The model under review builds one solid part; all positions refer to its coordinate system, in mm. A direction names the side the tool comes from. Coordinates: 2 decimals unless noted, no trailing zeros. Order: outer loops, then holes, each group sorted by start corner. A loop starts at its lowest first (then second) coordinate and runs counter-clockwise, first axis right, second up.
```python
from build123d import *

# Parameters (mm, degrees)
EXTRUDE_1_DEPTH     = 20
SKETCH_2_R          = 1.5
CUT_EXTRUDE_1_DEPTH = 4
SKETCH_3_R          = 2
CUT_EXTRUDE_2_DEPTH = 19
SKETCH_4_W          = 20
SKETCH_4_H          = 15
CUT_EXTRUDE_3_DEPTH = 1
SKETCH_5_W          = 20
SKETCH_5_H          = 23
CUT_EXTRUDE_4_DEPTH = 1


with BuildPart() as part:
    # 草图1 → 凸台-拉伸1 (new body)
    with BuildSketch(Plane(origin=(0, 0, 0), x_dir=(0, 0, -1), z_dir=(1, 0, 0))):
        Polygon((0, 0), (0, 25), (3, 25), (3, 3), (18, 3), (18, 0), align=None)
    extrude(amount=EXTRUDE_1_DEPTH)

    # 草图2 → 切除-拉伸1 (cut, through all)
    with BuildSketch(Plane(origin=(0, 3, 0), x_dir=(1, 0, 0), z_dir=(0, 1, 0))):
        with Locations((5.5, 8)):
            Circle(SKETCH_2_R)
        with Locations((14.5, 8)):
            Circle(SKETCH_2_R)
    extrude(amount=-CUT_EXTRUDE_1_DEPTH, mode=Mode.SUBTRACT)

    # 草图3 → 切除-拉伸2 (cut, through all)
    with BuildSketch(Plane.XY):
        with Locations((10, 16)):
            Circle(SKETCH_3_R)
    extrude(amount=-CUT_EXTRUDE_2_DEPTH, mode=Mode.SUBTRACT)

    # 草图4 → 切除-拉伸3 (cut)
    with BuildSketch(Plane(origin=(0, 3, 0), x_dir=(1, 0, 0), z_dir=(0, 1, 0))):
        with Locations((10, 10.5)):
            Rectangle(SKETCH_4_W, SKETCH_4_H)
    extrude(amount=-CUT_EXTRUDE_3_DEPTH, mode=Mode.SUBTRACT)

    # 草图5 → 切除-拉伸4 (cut)
    with BuildSketch(Plane(origin=(0, 0, -3), x_dir=(-1, 0, 0), z_dir=(0, 0, -1))):
        with Locations((-10, 13.5)):
            Rectangle(SKETCH_5_W, SKETCH_5_H)
    extrude(amount=-CUT_EXTRUDE_4_DEPTH, mode=Mode.SUBTRACT)


solid = part.part
```
(1) We need section A-A, the plane x = 14.5. Write out the cut boundary in (y, z), and give its area (3 significant figures).
A:
outline: (0, -18) - (2, -18) - (2, -9.5) - (0, -9.5) - close; (0, -6.5) - (2, -6.5) - (2, -2) - (25, -2) - (25, 0) - (0, 0) - close
area: 76.0 mm2
(2) We need section C-C, the plane y = 16. Write out the cut boundary in (x, z).
A:
outline: (0, -2) - (8, -2) - (8, 0) - (0, 0) - close; (12, -2) - (20, -2) - (20, 0) - (12, 0) - close
(3) Machinability: for faces 5 (the face through (10.1, 13.7, -2)), 6 (the face through (20, 7.9, -1.7)), which of the approach directions +Z, -Z, +X, -X, +Y, -Y give a long, thin tool a straight path to every point of the face, cutting with its end or side? Answer none if there is none.
A:
face 5: -Z, +X, -X, +Y
face 6: +Z, -Z, +X, +Y, -Y
(4) Wall thickness on probe 1 along X at (y, z) = (1.4, -8); probe 2 along Z at (x, y) = (5.5, 0.6); probe 3 along Y at (x, z) = (10, -0.5): over which ranges is each line inside the solid? List them lowest first.
A:
probe 1: x = 0 to 4, 7 to 13, 16 to 20
probe 2: z = -18 to -9.5, -6.5 to 0
probe 3: y = 0 to 14, 18 to 25
(5) We need section B-B, the plane z = -8. Write out the cut boundary in (x, y).
A:
outline: (0, 0) - (4, 0) - (4, 2) - (0, 2) - close; (7, 0) - (13, 0) - (13, 2) - (7, 2) - close; (16, 0) - (20, 0) - (20, 2) - (16, 2) - close
(6) We need section D-D, the plane z = -1.5. Write out the cut boundary in (x, y).
A:
outline: (0, 0) - (20, 0) - (20, 25) - (0, 25) - close; hole circle Ø4 at (10, 16)
(7) For pin 1 Ø1.5 at (y, z) = (3, -5) entering from -X; pin 2 Ø6 at (x, y) = (10, 18) entering from -Z; pin 3 Ø6 at (x, z) = (17.5, -15.5) entering from +Y, all flat-tipped, find the tip position at first contact; note any pin that passes through.
A:
pin 1: passes through
pin 2: stops at z = -2
pin 3: stops at y = 2
(8) Draft analysis for pull direction Y (two halves, no side actions). For faces 1 (the face through (10, 0, -9)), 2 (the face through (10, 25, -1)), 3 (the face through (10, 1, -18)), 4 (the face through (10, 18, -1)), state which applies: released by +Y, released by -Y, zero draft, split by the parting line, or undercut.
A:
face 1: released by -Y
face 2: released by +Y
face 3: zero draft
face 4: undercut
